from build123d import *

# Parameters (mm, degrees)
ESQUISSE1_W             = 32.5
ESQUISSE1_H             = 30
BOSS_EXTRU_1_DEPTH      = 2
ESQUISSE1_4_W           = 25
ESQUISSE1_4_H           = 27
ESQUISSE1_4_W_2         = 24
ESQUISSE1_4_H_2         = 26
BOSS_EXTRU_2_DEPTH      = 15
ESQUISSE6_R             = 3.5
ENL_V_MAT_EXTRU_2_DEPTH = 0.5
ESQUISSE5_R             = 3.5
ENL_V_MAT_EXTRU_3_DEPTH = 0.5


with BuildPart() as part:
    # Esquisse1 → Boss.-Extru.1 (new body)
    with BuildSketch(Plane(origin=(0, 0, 0), x_dir=(1, 0, 0), z_dir=(0, 1, 0))):
        with Locations((-4.171052632, 10.289473684)):
            Rectangle(ESQUISSE1_W, ESQUISSE1_H)
    extrude(amount=BOSS_EXTRU_1_DEPTH)

    # Esquisse1_4 → Boss.-Extru.2 (add)
    with BuildSketch(Plane(origin=(0, 0, 0), x_dir=(1, 0, 0), z_dir=(0, 1, 0))):
        with Locations((-7.921052632, 10.289473684)):
            Rectangle(ESQUISSE1_4_W, ESQUISSE1_4_H)
        with Locations((-7.921052632, 10.289473684)):
            Rectangle(ESQUISSE1_4_W_2, ESQUISSE1_4_H_2, mode=Mode.SUBTRACT)
    extrude(amount=BOSS_EXTRU_2_DEPTH)

    # Esquisse6 → Enl_v. mat.-Extru.2 (cut)
    with BuildSketch(Plane.XY.offset(3.210526316)):
        with Locations((-14.421052632, 8.5)):
            Circle(ESQUISSE6_R)
    extrude(amount=-ENL_V_MAT_EXTRU_2_DEPTH, mode=Mode.SUBTRACT)

    # Esquisse5 → Enl_v. mat.-Extru.3 (cut)
    with BuildSketch(Plane(origin=(0, 0, -23.789473684), x_dir=(-1, 0, 0), z_dir=(0, 0, -1))):
        with Locations(Location((14.421052632, 8.5, 0), (0, 0, 180))):
            Circle(ESQUISSE5_R)
    extrude(amount=-ENL_V_MAT_EXTRU_3_DEPTH, mode=Mode.SUBTRACT)


solid = part.part
Could you check a few things on this model? Use its own coordinates, in mm. A direction names the side the tool comes from. Coordinates: 2 decimals unless noted, no trailing zeros. Loops run counter-clockwise (first coordinate to the right, second up) from the corner with the lowest first, then second, coordinate; pieces in that order, holes last.
1. Imagine slicing it at A-A (y = 4). Please give me the cut outline in (x, z).
2. For P1, Ø3, axis at x = 0, z = -19.5, coming from the +Y side; P2, Ø4, axis at y = 5, z = -11.5, coming from the +X side; P3, Ø4, axis at x = -9.5, y = 11, coming from the -Z side; P4, Ø12, axis at x = 5.5, z = -6.5, coming from the +Y side, each with a flat end and sliding along its axis, tell me the tip position at first contact or that it passes through.
3. For faces 4 (the face through (-8, 2, -10)), 5 (the face through (-8, 8, 3.211)), 6 (the face through (4.579, 8, -10)), 7 (the face through (-8, 8, -23.789)), 8 (the face through (12.079, 1, -10)), which set-ups out of +Z, -Z, +X, -X, +Y, -Y let a thin tool reach every point of the face, with its end or its side?
4. Imagine slicing it at B-B (y = 8.5). Please give me the cut outline in (x, z), and give its area (3 significant figures).
5. I need wall thicknesses on L1, parallel to Z at x = 0.5, y = 5.5; L2, parallel to X at y = 12.5, z = -17.25; L3, parallel to Y at x = 3, z = -5.75. Which ranges of each line are inside material? Lowest first, please.
6. Imagine slicing it at D-D (z = -12.75). Please give me the cut outline in (x, y), and give its area (3 significant figures).
7. Imagine slicing it at C-C (x = -9). Please give me the cut outline in (y, z).
8. We'd pull the mould along Y, two halves only. Please class faces 1 (the face through (-19.921, 8, -10)), 2 (the face through (-15.18, 5.083, 2.964)), 3 (the face through (-4, 0, -10)): released by +Y, released by -Y, zero draft, split by the parting line, or undercut.
Computed values:
1. outline: (-20.42, -23.79) - (4.58, -23.79) - (4.58, 3.21) - (-20.42, 3.21) - close; hole (-19.92, -23.29) - (4.08, -23.29) - (4.08, 2.71) - (-19.92, 2.71) - close
2. P1: stops at y = 2
2. P2: stops at x = 4.58
2. P3: stops at z = -23.79
2. P4: stops at y = 15
3. face 4: +Y
3. face 5: +Z, +X, -X, +Y
3. face 6: +Z, -Z, +X, +Y
3. face 7: -Z, +X, -X, +Y
3. face 8: +Z, -Z, +X, +Y, -Y
4. outline: (-20.42, -23.79) - (-17.92, -23.79) - (-17.92, -23.29) - (-19.92, -23.29) - (-19.92, 2.71) - (-17.92, 2.71) - (-17.92, 3.21) - (-20.42, 3.21) - close; (-10.92, -23.79) - (4.58, -23.79) - (4.58, 3.21) - (-10.92, 3.21) - (-10.92, 2.71) - (4.08, 2.71) - (4.08, -23.29) - (-10.92, -23.29) - close
4. area: 44.0 mm2
5. L1: z = -23.79 to -23.29, 2.71 to 3.21
5. L2: x = -20.42 to -19.92, 4.08 to 4.58
5. L3: y = 0 to 2
6. outline: (-20.42, 0) - (12.08, 0) - (12.08, 2) - (4.58, 2) - (4.58, 15) - (4.08, 15) - (4.08, 2) - (-19.92, 2) - (-19.92, 15) - (-20.42, 15) - close
6. area: 78.0 mm2
7. outline: (0, -25.29) - (2, -25.29) - (2, -23.79) - (15, -23.79) - (15, -23.29) - (2, -23.29) - (2, 2.71) - (15, 2.71) - (15, 3.21) - (2, 3.21) - (2, 4.71) - (0, 4.71) - close
8. face 1: zero draft
8. face 2: undercut
8. face 3: released by -Y
